Print and shaded views of the part. All mm, measured from the part's lowest x, y and z. A direction names the side the tool comes from. Give positions to 0.01 mm unless a question says otherwise; leave off trailing zeros. Loops run counter-clockwise (first coordinate to the right, second up) from the corner with the lowest first, then second, coordinate; pieces in that order, holes last.
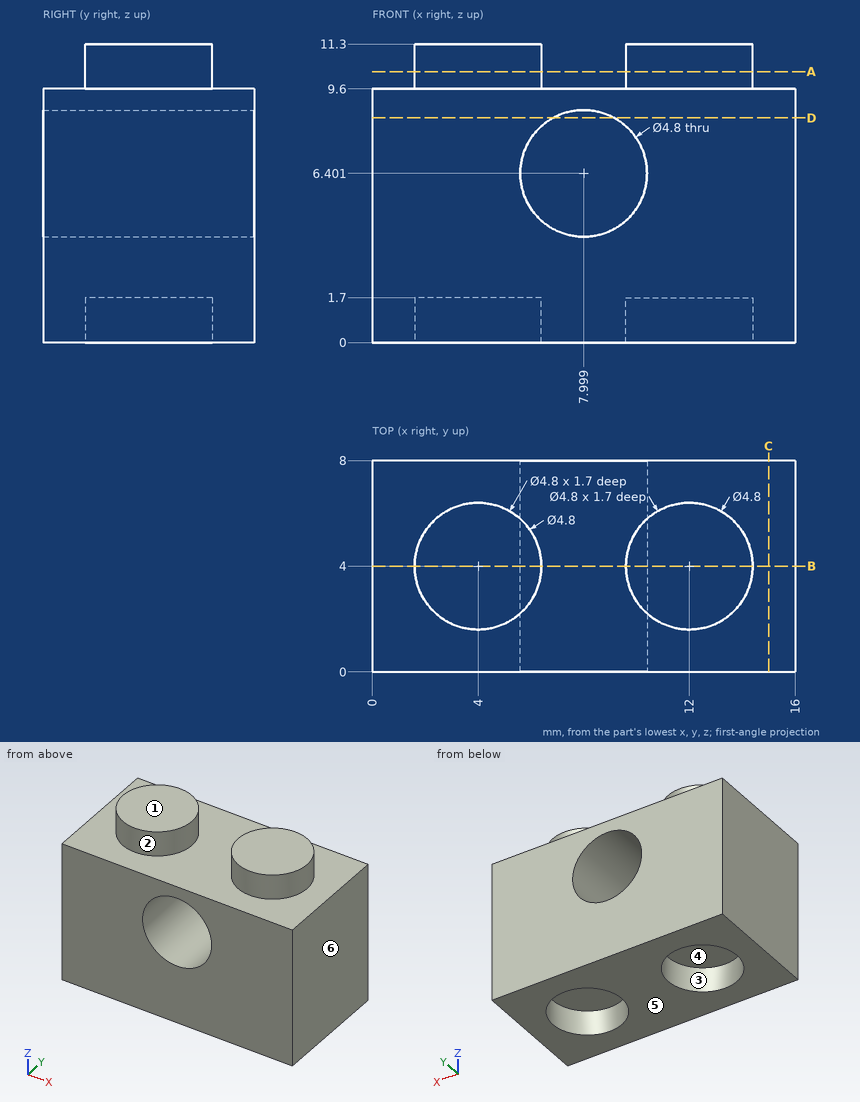
1. Saw through at D-D, the plane z = 8.5. List the corners of the cut face in (x, y), and give its area (3 significant figures).
Responses:
outline: (0, 0) - (6.84, 0) - (6.84, 8) - (0, 8) - close; (9.16, 0) - (16, 0) - (16, 8) - (9.16, 8) - close
area: 109 mm2
2. Saw through at B-B, the plane y = 4. List the corners of the cut face in (x, z), and give its area (4 significant figures).
Responses:
outline: (0, 0) - (1.6, 0) - (1.6, 1.7) - (6.4, 1.7) - (6.4, 0) - (9.6, 0) - (9.6, 1.7) - (14.4, 1.7) - (14.4, 0) - (16, 0) - (16, 9.6) - (14.4, 9.6) - (14.4, 11.3) - (9.6, 11.3) - (9.6, 9.6) - (6.4, 9.6) - (6.4, 11.3) - (1.6, 11.3) - (1.6, 9.6) - (0, 9.6) - close; hole circle Ø4.8 at (8, 6.4)
area: 135.5 mm2
3. Probe line 1 along Y through (x, z) = (12, 1.4); line 2 along X through (y, z) = (2.5, 1.5); line 3 along X through (y, z) = (3.25, 1.5). List the from-to ranges inside material, lowest first.
Responses:
line 1: y = 0 to 1.6, 6.4 to 8
line 2: x = 0 to 2.13, 5.87 to 10.13, 13.87 to 16
line 3: x = 0 to 1.72, 6.28 to 9.72, 14.28 to 16
4. Saw through at C-C, the plane x = 15. List the corners of the cut face in (y, z).
Responses:
outline: (0, 0) - (8, 0) - (8, 9.6) - (0, 9.6) - close
5. Tool access for the marked faces 1, 2 and 3: list every direction of +Z, -Z, +X, -X, +Y, -Y with a clear straight run to the whole face (end or side of a thin tool).
Responses:
face 1: +Z, +X, -X, +Y, -Y
face 2: +Z
face 3: -Z
6. Pull direction X, two halves, no side cores. Call the marked faces 4, 5 and 6: released by +X, released by -X, zero draft, split by the parting line, or undercut.
Responses:
face 4: undercut
face 5: zero draft
face 6: released by +X
7. Drop flat-ended pins along their axis: pin 1 (3 mm diameter, centred on x = 10, y = 6, fed in from -Z); pin 2 (2.5 mm diameter, centred on x = 4, y = 5, fed in from -Z). Give the stop position or say it passes through.
Responses:
pin 1: stops at z = 0
pin 2: stops at z = 1.7
8. Saw through at A-A, the plane z = 10.25. List the corners of the cut face in (x, y), and give its area (3 significant figures).
Responses:
outline: circle Ø4.8 at (4, 4); circle Ø4.8 at (12, 4)
area: 36.2 mm2
